Input: part model. Units: mm. Frame: model coordinates. Face numbers are marked on the shaded views. A direction names the side the tool comes from. Give positions to 0.01 mm unless a question says otherwise; leave off trailing zeros. Write each loop counter-clockwise with the first axis right and the second up, starting at its lowest first coordinate (ties: lowest second). Pieces come first, ordered by that corner, then holes. Notation, with made-up numbers: (78, 78.25) -> (96, 78.25) arc R6 cw to (96, 83.25) -> close; hole circle Ø11 at (-23, 49.25). An arc over 180 degrees is marked (long way). Return JSON: item names as keys, results as strings. Group by question number.
Item 1: Set-up query: the marked faces 1, 2 and 3. Return all of +Z, -Z, +X, -X, +Y, -Y with unobstructed straight access to the full face (end or side cutting, diameter ignored); none if empty.
Item 2: Section A-A, the plane x = -11. Return loops of the section in (y, z).
Item 3: Line query: line 1 (Z direction, x = 16.95, y = 21); line 2 (Y direction, x = 16, z = -16); line 3 (X direction, y = -18, z = -52). Output: solid intervals per line, ascending. Write a range as [from, to].
Item 4: Section B-B, the plane z = -69.5. Return loops of the section in (x, y).
Item 5: Section C-C, the plane z = -60. Return loops of the section in (x, y), then the cut area to 3 significant figures.
Item 6: Pin query (flat end, axial travel): P1, Ø3.5, axis at y = -15.5, z = -47.5, coming from the +X side; P2, Ø1, axis at y = -12.5, z = -66, coming from the -X side; P3, Ø0.8, axis at x = 18, y = 20.5, coming from the +Z side; P4, Ø0.5, axis at x = 18, y = 20.5, coming from the -Z side. Return the tip coordinate at first contact, or that it passes through.
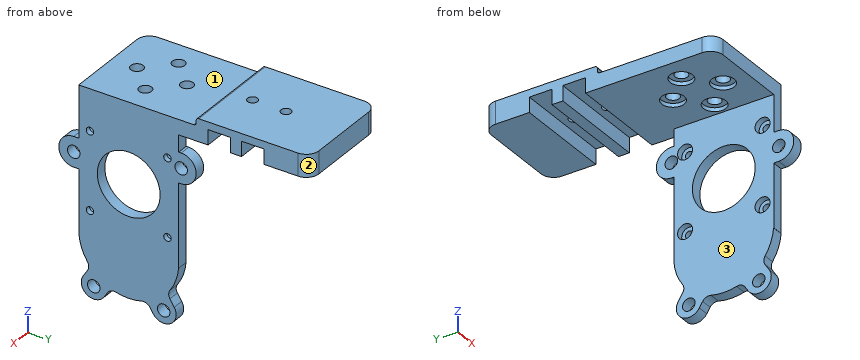
from build123d import *

# Parameters (mm, degrees)
SKETCH2_W            = 40
SKETCH2_H            = 40
SKETCH2_R            = 2.5
BOSS_EXTRUDE1_DEPTH  = 6
SKETCH3_W            = 4.5
SKETCH3_H            = 40
BOSS_EXTRUDE2_DEPTH  = 52
CUT_EXTRUDE1_REACH   = 6.5
SKETCH4_R            = 12.573151632
SKETCH4_R_2          = 1.5
SKETCH5_R            = 4.5
CUT_EXTRUDE2_DEPTH   = 1.5
SKETCH6_R            = 3
CUT_EXTRUDE3_DEPTH   = 2.5
FILLET1_R            = 5
SKETCH11_R           = 2.5
BOSS_EXTRUDE6_DEPTH  = 4.5
FILLET2_R            = 3
SKETCH9_R            = 2.5
BOSS_EXTRUDE15_DEPTH = 4.5
SKETCH24_R           = 2.5
CUT_EXTRUDE11_DEPTH  = 4.5
SKETCH15_R           = 3
CUT_EXTRUDE12_DEPTH  = 2.5
SKETCH25_W           = 40
SKETCH25_H           = 9
BOSS_EXTRUDE16_DEPTH = 52.75
SKETCH28_W           = 40
SKETCH28_H           = 2
CUT_EXTRUDE15_DEPTH  = 3
SKETCH33_W           = 40
SKETCH33_H           = 5
CUT_EXTRUDE18_DEPTH  = 3
FILLET7_R            = 1
FILLET8_R            = 5
SKETCH31_W           = 40
SKETCH31_H           = 9.0424
CUT_EXTRUDE16_DEPTH  = 6
SKETCH32_R           = 2
CUT_EXTRUDE17_DEPTH  = 4


with BuildPart() as part:
    # Sketch2 → Boss-Extrude1 (new body)
    with BuildSketch(Plane.XY):
        Rectangle(SKETCH2_W, SKETCH2_H)
        with Locations((0, 10)):
            Circle(SKETCH2_R, mode=Mode.SUBTRACT)
        with Locations((0, -10)):
            Circle(SKETCH2_R, mode=Mode.SUBTRACT)
        with Locations((-10, 0)):
            Circle(SKETCH2_R, mode=Mode.SUBTRACT)
        with Locations((10, 0)):
            Circle(SKETCH2_R, mode=Mode.SUBTRACT)
    extrude(amount=-BOSS_EXTRUDE1_DEPTH)

    # Sketch3 → Boss-Extrude2 (add)
    with BuildSketch(Plane(origin=(0, 0, -6), x_dir=(-1, 0, 0), z_dir=(0, 0, -1))):
        with Locations((-17.75, 0)):
            Rectangle(SKETCH3_W, SKETCH3_H)
    extrude(amount=BOSS_EXTRUDE2_DEPTH)

    # Sketch4 → Cut-Extrude1 (cut, up to next)
    with BuildSketch(Plane.ZY.offset(-15.5), mode=Mode.PRIVATE) as cut_extrude1_sk1:
        with Locations((-32, 0)):
            Circle(SKETCH4_R)
    cut_extrude1_tool1 = extrude(cut_extrude1_sk1.sketch, amount=-CUT_EXTRUDE1_REACH, mode=Mode.PRIVATE) & part.part
    add(cut_extrude1_tool1.solids().sort_by_distance((15.5, 0, -32))[0], mode=Mode.SUBTRACT)
    # Sketch4 → Cut-Extrude1 (cut, up to next)
    with BuildSketch(Plane.ZY.offset(-15.5), mode=Mode.PRIVATE) as cut_extrude1_sk2:
        with Locations((-16.5, 15.5)):
            Circle(SKETCH4_R_2)
    cut_extrude1_tool2 = extrude(cut_extrude1_sk2.sketch, amount=-CUT_EXTRUDE1_REACH, mode=Mode.PRIVATE) & part.part
    add(cut_extrude1_tool2.solids().sort_by_distance((15.5, 15.5, -16.5))[0], mode=Mode.SUBTRACT)
    # Sketch4 → Cut-Extrude1 (cut, up to next)
    with BuildSketch(Plane.ZY.offset(-15.5), mode=Mode.PRIVATE) as cut_extrude1_sk3:
        with Locations((-16.5, -15.5)):
            Circle(SKETCH4_R_2)
    cut_extrude1_tool3 = extrude(cut_extrude1_sk3.sketch, amount=-CUT_EXTRUDE1_REACH, mode=Mode.PRIVATE) & part.part
    add(cut_extrude1_tool3.solids().sort_by_distance((15.5, -15.5, -16.5))[0], mode=Mode.SUBTRACT)
    # Sketch4 → Cut-Extrude1 (cut, up to next)
    with BuildSketch(Plane.ZY.offset(-15.5), mode=Mode.PRIVATE) as cut_extrude1_sk4:
        with Locations((-47.5, -15.5)):
            Circle(SKETCH4_R_2)
    cut_extrude1_tool4 = extrude(cut_extrude1_sk4.sketch, amount=-CUT_EXTRUDE1_REACH, mode=Mode.PRIVATE) & part.part
    add(cut_extrude1_tool4.solids().sort_by_distance((15.5, -15.5, -47.5))[0], mode=Mode.SUBTRACT)
    # Sketch4 → Cut-Extrude1 (cut, up to next)
    with BuildSketch(Plane.ZY.offset(-15.5), mode=Mode.PRIVATE) as cut_extrude1_sk5:
        with Locations((-47.5, 15.5)):
            Circle(SKETCH4_R_2)
    cut_extrude1_tool5 = extrude(cut_extrude1_sk5.sketch, amount=-CUT_EXTRUDE1_REACH, mode=Mode.PRIVATE) & part.part
    add(cut_extrude1_tool5.solids().sort_by_distance((15.5, 15.5, -47.5))[0], mode=Mode.SUBTRACT)

    # Sketch5 → Cut-Extrude2 (cut)
    with BuildSketch(Plane(origin=(0, 0, -6), x_dir=(-1, 0, 0), z_dir=(0, 0, -1))):
        with Locations((0, 10)):
            Circle(SKETCH5_R)
        with Locations((10, 0)):
            Circle(SKETCH5_R)
        with Locations((0, -10)):
            Circle(SKETCH5_R)
        with Locations((-10, 0)):
            Circle(SKETCH5_R)
    extrude(amount=-CUT_EXTRUDE2_DEPTH, mode=Mode.SUBTRACT)

    # Sketch6 → Cut-Extrude3 (cut)
    with BuildSketch(Plane.ZY.offset(-15.5)):
        with Locations((-16.5, 15.5)):
            Circle(SKETCH6_R)
        with Locations((-47.5, 15.5)):
            Circle(SKETCH6_R)
        with Locations((-47.5, -15.5)):
            Circle(SKETCH6_R)
        with Locations((-16.5, -15.5)):
            Circle(SKETCH6_R)
    extrude(amount=-CUT_EXTRUDE3_DEPTH, mode=Mode.SUBTRACT)

    # Fillet1
    fillet1_edges = [part.edges().sort_by_distance(p)[0] for p in [
        (-20, -20, -3),
    ]]
    fillet(fillet1_edges, radius=FILLET1_R)

    # Sketch11 → Boss-Extrude6 (add)
    with BuildSketch(Plane.ZY.offset(-15.5)):
        with BuildLine():
            Line((-58, -19.943670675), (-58, 19.943670675))
            ThreePointArc((-58, 19.943670675), (-64.026515977, 18.5297479), (-69.332027993, 15.34076457))
            ThreePointArc((-69.332027993, 15.34076457), (-72.76360296, 11.640241353), (-75.159610133, 7.198538025))
            ThreePointArc((-75.159610133, 7.198538025), (-76.5, 0), (-75.159610133, -7.198538025))
            ThreePointArc((-75.159610133, -7.198538025), (-72.76360296, -11.640241353), (-69.332027993, -15.34076457))
            ThreePointArc((-69.332027993, -15.34076457), (-64.026515977, -18.5297479), (-58, -19.943670675))
        make_face()
        with BuildLine():
            ThreePointArc((-75.159610133, 7.198538025), (-72.76360296, 11.640241353), (-69.332027993, 15.34076457))
            Line((-69.332027993, 15.34076457), (-73.799349609, 18.20790773))
            ThreePointArc((-73.799349609, 18.20790773), (-80.70790773, 16.700650391), (-79.200650391, 9.79209227))
            Line((-79.200650391, 9.79209227), (-75.159610133, 7.198538025))
        make_face()
        with Locations((-76.5, 14)):
            Circle(SKETCH11_R, mode=Mode.SUBTRACT)
        with BuildLine():
            Line((-73.799349609, -18.20790773), (-69.332027993, -15.34076457))
            ThreePointArc((-69.332027993, -15.34076457), (-72.76360296, -11.640241353), (-75.159610133, -7.198538025))
            Line((-75.159610133, -7.198538025), (-79.200650391, -9.79209227))
            ThreePointArc((-79.200650391, -9.79209227), (-80.70790773, -16.700650391), (-73.799349609, -18.20790773))
        make_face()
        with Locations((-76.5, -14)):
            Circle(SKETCH11_R, mode=Mode.SUBTRACT)
    extrude(amount=-BOSS_EXTRUDE6_DEPTH)

    # Fillet2
    fillet2_edges = [part.edges().sort_by_distance(p)[0] for p in [
        (17.75, -15.34076457, -69.332027993),
        (17.75, -7.198538025, -75.159610133),
        (17.75, 7.198538025, -75.159610133),
        (17.75, 15.34076457, -69.332027993),
    ]]
    fillet(fillet2_edges, radius=FILLET2_R)

    # Sketch9 → Boss-Extrude15 (add)
    with BuildSketch(Plane.ZY.offset(-15.5)):
        with BuildLine():
            Line((-32.75, -22), (-32.75, -18.434411342))
            Line((-32.75, -18.434411342), (-20.75, -18.434411342))
            Line((-20.75, -18.434411342), (-20.75, -22))
            ThreePointArc((-20.75, -22), (-26.75, -28), (-32.75, -22))
        make_face()
        with Locations((-26.75, -22)):
            Circle(SKETCH9_R, mode=Mode.SUBTRACT)
        with BuildLine():
            Line((-24.75, 21), (-24.75, 17.603718698))
            Line((-24.75, 17.603718698), (-12.75, 17.603718698))
            Line((-12.75, 17.603718698), (-12.75, 21))
            ThreePointArc((-12.75, 21), (-18.75, 27), (-24.75, 21))
        make_face()
        with Locations((-18.75, 21)):
            Circle(SKETCH9_R, mode=Mode.SUBTRACT)
    extrude(amount=-BOSS_EXTRUDE15_DEPTH)

    # Sketch24 → Cut-Extrude11 (cut)
    with BuildSketch(Plane.ZY.offset(-15.5)):
        with Locations((-18.75, 21)):
            Circle(SKETCH24_R)
        with Locations((-26.75, -22)):
            Circle(SKETCH24_R)
    extrude(amount=-CUT_EXTRUDE11_DEPTH, mode=Mode.SUBTRACT)

    # Sketch15 → Cut-Extrude12 (cut)
    with BuildSketch(Plane.ZY.offset(-15.5)):
        with Locations((-16.5, 15.5)):
            Circle(SKETCH15_R)
    extrude(amount=-CUT_EXTRUDE12_DEPTH, mode=Mode.SUBTRACT)

    # Sketch25 → Boss-Extrude16 (add)
    with BuildSketch(Plane(origin=(0, 20, 0), x_dir=(1, 0, 0), z_dir=(0, 1, 0))):
        with Locations((0, 1.5)):
            Rectangle(SKETCH25_W, SKETCH25_H)
    extrude(amount=BOSS_EXTRUDE16_DEPTH)

    # Sketch28 → Cut-Extrude15 (cut)
    with BuildSketch(Plane.XY.offset(3)):
        with Locations((0, 21)):
            Rectangle(SKETCH28_W, SKETCH28_H)
    extrude(amount=-CUT_EXTRUDE15_DEPTH, mode=Mode.SUBTRACT)

    # Sketch33 → Cut-Extrude18 (cut)
    with BuildSketch(Plane.XY.offset(3)):
        with Locations((0, 24.5)):
            Rectangle(SKETCH33_W, SKETCH33_H)
    extrude(amount=-CUT_EXTRUDE18_DEPTH, mode=Mode.SUBTRACT)

    # Fillet7
    fillet7_edges = [part.edges().sort_by_distance(p)[0] for p in [
        (0, 27, 3),
        (0, 27, 0),
    ]]
    fillet(fillet7_edges, radius=FILLET7_R)

    # Fillet8
    fillet8_edges = [part.edges().sort_by_distance(p)[0] for p in [
        (20, 72.75, -1.5),
        (-20, 72.75, -1.5),
    ]]
    fillet(fillet8_edges, radius=FILLET8_R)

    # Sketch31 → Cut-Extrude16 (cut)
    with BuildSketch(Plane(origin=(0, 0, -6), x_dir=(-1, 0, 0), z_dir=(0, 0, -1))):
        with Locations((0, 36.2712)):
            Rectangle(SKETCH31_W, SKETCH31_H)
        with Locations((0, 49.6636)):
            Rectangle(SKETCH31_W, SKETCH31_H)
    extrude(amount=-CUT_EXTRUDE16_DEPTH, mode=Mode.SUBTRACT)

    # Sketch32 → Cut-Extrude17 (cut, through all)
    with BuildSketch(Plane(origin=(0, 0, 0), x_dir=(-1, 0, 0), z_dir=(0, 0, -1))):
        with Locations((0, 49.6636)):
            Circle(SKETCH32_R)
        with Locations((0, 36.2712)):
            Circle(SKETCH32_R)
    extrude(amount=-CUT_EXTRUDE17_DEPTH, mode=Mode.SUBTRACT)


solid = part.part
Answer below:
{
 "1": {"face 1": "+Z, +X, -X, -Y", "face 2": "+Z, -Z, +X, +Y", "face 3": "-Z, -X, +Y, -Y"},
 "2": {"outline": "(-20, -6) -> (-4.39, -6) -> (-4.39, -4.5) -> (-2.29, -4.5) -> (-2.29, 0) -> (-20, 0) -> close; (2.29, -4.5) -> (4.39, -4.5) -> (4.39, -6) -> (31.75, -6) -> (31.75, 0) -> (40.79, 0) -> (40.79, -6) -> (45.14, -6) -> (45.14, 0) -> (54.18, 0) -> (54.18, -6) -> (72.75, -6) -> (72.75, 3) -> (28, 3) arc R1 ccw to (27, 2) -> (27, 1) arc R1 cw to (26, 0) -> (2.29, 0) -> close"},
 "3": {"line 1": "z = [-24.75, -21.25], [-16.25, -12.75], [-6, 0]", "line 2": "y = [-20, -18.46], [-12.54, 12.54], [18.46, 26.33]", "line 3": "x = [15.5, 20]"},
 "4": {"outline": "(15.5, -15.99) -> (20, -15.99) -> (20, 15.99) -> (15.5, 15.99) -> close"},
 "5": {"outline": "(15.5, -19.69) -> (20, -19.69) -> (20, 19.69) -> (15.5, 19.69) -> close", "area": "177 mm2"},
 "6": {"P1": "stops at x = 20", "P2": "stops at x = 15.5", "P3": "stops at z = 0", "P4": "stops at z = -24.75"}
}
